from build123d import *

# Parameters (mm, degrees)
SKETCH_R          = 5.6
SKETCH_R_2        = 4
PAD_DEPTH         = 8
SKETCH001_R       = 1.5
POCKET_DEPTH      = 100
POCKET_DEPTH_BACK = 100


with BuildPart() as part:
    # Sketch → Pad (new body)
    with BuildSketch(Plane.XY):
        with BuildLine():
            ThreePointArc((-12.5, 0), (0, -12.5), (12.5, 0))
            Line((12.5, 0), (12.5, 23))
            Line((-12.5, 23), (12.5, 23))
            Line((-12.5, 0), (-12.5, 23))
        make_face()
        Circle(SKETCH_R, mode=Mode.SUBTRACT)
        with Locations((0, 17)):
            Circle(SKETCH_R_2, mode=Mode.SUBTRACT)
    extrude(amount=PAD_DEPTH)

    # Sketch001 → Pocket (cut, two sides)
    with BuildSketch(Plane.YZ) as pocket_sk:
        with Locations((0, 4)):
            Circle(SKETCH001_R)
    extrude(amount=-POCKET_DEPTH, mode=Mode.SUBTRACT)
    extrude(pocket_sk.sketch, amount=POCKET_DEPTH_BACK, mode=Mode.SUBTRACT)


solid = part.part
Design review of the part built by this model. Coordinates are the model's own, in mm. Round coordinates to 2 decimals unless told otherwise and drop trailing zeros. Order: outer loops, then holes, each group sorted by start corner. A loop starts at its lowest first (then second) coordinate and runs counter-clockwise, first axis right, second up. Notation, with made-up numbers: M 48.5,61 L 55.5,61 A17 ccw 55.5,77 Z; hole C 48.5,30.5 d1. An arc over 180 degrees is marked long. Answer as CSV lines item,"result". Start each with the question number.
1) Wall thickness on line 1 along Y through (x, z) = (-0.5, 5); line 2 along Y through (x, z) = (-3.5, 5.5); line 3 along Z through (x, y) = (7.25, 0): over which ranges is each line inside the solid? List them lowest first. Write a range as [from, to].
2) Add section C-C (x = 0). Give the boundary of the cut face in (y, z), then the cut area to 3 significant figures.
3) Add section A-A (y = 17). Give the boundary of the cut face in (x, z).
4) Add section B-B (z = 3.25). Give the boundary of the cut face in (x, y).
5) The part is to be moulded in two halves that separate along Y. For faces 1 (the face through (12.5, 11, 4)), 2 (the face through (-0.521, 20.966, 3.944)), 3 (the face through (8.898, 0.806, 5.265)), 4 (the face through (0, 23, 4)), say which applies: +Y half, -Y half, draft (parallel to the pull), parting line (faces both ways), or undercut.
6) Add section D-D (z = 7). Give the boundary of the cut face in (x, y), then the cut area to 3 significant figures.
Resolved:
1,line 1,"[-12.49, -5.58], [5.58, 13.03], [20.97, 23]"
1,line 2,"[-12, -4.37], [4.37, 15.06], [18.94, 23]"
1,line 3,"[0, 2.5], [5.5, 8]"
2,outline,"M -12.5,0 L -5.6,0 L -5.6,8 L -12.5,8 Z; M 5.6,0 L 13,0 L 13,8 L 5.6,8 Z; M 21,0 L 23,0 L 23,8 L 21,8 Z"
2,area,"130 mm^2"
3,outline,"M -12.5,0 L -4,0 L -4,8 L -12.5,8 Z; M 4,0 L 12.5,0 L 12.5,8 L 4,8 Z"
4,outline,"M -12.5,1.3 L -5.45,1.3 A5.6 cw 5.45,1.3 L 12.5,1.3 L 12.5,23 L -12.5,23 Z; M -12.43,-1.3 A12.5 ccw 12.43,-1.3 L 5.45,-1.3 A5.6 cw -5.45,-1.3 Z; hole C 0,17 d8"
5,face 1,"draft"
5,face 2,"undercut"
5,face 3,"undercut"
5,face 4,"+Y half"
6,outline,"M -12.5,0 A12.5 ccw 12.5,0 L 12.5,23 L -12.5,23 Z; hole C 0,0 d11.2; hole C 0,17 d8"
6,area,"672 mm^2"
